Source: CAD feature listing. Evaluate the final solid. Frame: model axes, mm. A direction names the side the tool comes from. Give positions to 0.01 mm unless a question says otherwise; leave off trailing zeros. Order: outer loops, then holes, each group sorted by start corner. A loop starts at its lowest first (then second) coordinate and runs counter-clockwise, first axis right, second up. Notation, with made-up numbers: (62.5, 18) -> (81.5, 18) arc R25 cw to (81.5, 37) -> close; hole circle Ø4 at (-33, 62.5). An arc over 180 degrees is marked (long way). Answer in a Markdown table with one row per item.
Autodesk Inventor part; units mm, degrees
ref_plane "YZ Plane" through (0, 0, 0) normal (1, 0, 0) x (0, 1, 0)
ref_plane "XZ Plane" through (0, 0, 0) normal (0, 1, 0) x (-1, 0, 0)
ref_plane "XY Plane" through (0, 0, 0) normal (0, 0, 1) x (1, 0, 0)
sketch "Sketch1" plane through (0, 0, 0) normal (0, 0, 1) x (1, 0, 0)
  circle A0 centre (10.5, -1.5) radius 0.95
  circle A1 centre (-10.5, -1.5) radius 0.95
  line L0 (14, 9) -> (-14, 9)
  line L1 (-14, 9) -> (-14, -9)
  line L2 (-14, -9) -> (-7.5, -9)
  line L3 (-7.5, -9) -> (-7.5, -1.5)
  arc A2 (7.5, -1.5) -> (-7.5, -1.5) centre (0, -1.5) ccw
  line L4 (7.5, -1.5) -> (7.5, -9)
  line L5 (7.5, -9) -> (14, -9)
  line L6 (14, -9) -> (14, 9)
  line L7 (-7.5, -9) -> (7.5, -9)
  point P0 (0, 0)
extrude "Extrusion1" add sketch "Sketch1" along normal blind 3
sketch "Sketch2" plane through (0, 0, 3) normal (0, 0, 1) x (1, 0, 0)
  circle A0 centre (0, -1.5) radius 3
  circle A1 centre (0, -1.5) radius 2.95
  point P0 (0, 0)
  dimension "d4" = 5.9
extrude "Extrusion2" add sketch "Sketch2" along normal blind 5 contours A1
sketch "Sketch3" plane through (0, -1.5, 8) normal (0, 0, 1) x (1, 0, 0)
  circle A0 centre (0, 0) radius 2.95
  circle A1 centre (0, 0) radius 1.75
  point P0 (0, 1.5)
  dimension "d7" = 3.5
extrude "Extrusion3" cut sketch "Sketch3" against normal blind 8 contours A1
sketch "Sketch4" plane through (0, 0, 3) normal (0, 0, 1) x (1, 0, 0)
  circle A0 centre (0, -1.5) radius 2.95
  line L0 (14, -9) -> (14, 9)
  line L1 (14, 9) -> (-14, 9)
  line L2 (-14, 9) -> (-14, -9)
  line L3 (-14, -9) -> (14, -9)
  circle A1 centre (10.5, -1.5) radius 0.95
  circle A2 centre (-10.5, -1.5) radius 0.95
  line L4 (-5, -2) -> (-5, -1)
  line L5 (-5, -1) -> (5, -1)
  line L6 (5, -1) -> (5, -2)
  line L7 (5, -2) -> (-5, -2)
  line L8 (-5, -2) -> (5, -1) construction
  line L9 (-5, -1) -> (5, -2) construction
  point P0 (0, 0)
  dimension "d10" = 1
  dimension "d11" = 10
extrude "Extrusion4" cut sketch "Sketch4" along normal up to surface (5 mm away) contours A0 L7 L5 | A0 L5 L6 L7 | A0 L7 L4 L5
fillet "Fillet1" radius 0.5 4 edges at (2.2922, -2, 3) (-2.2922, -2, 3) (2.2922, -1, 3) (-2.2922, -1, 3)
sketch "Sketch5" plane through (0, 0, 3) normal (0, 0, 1) x (1, 0, 0)
  arc A0 (2.95, -1.5) -> (-2.95, -1.5) centre (0, -1.5) ccw
  arc A1 (-2.95, -1.5) -> (2.95, -1.5) centre (0, -1.5) ccw
  line L0 (14, -9) -> (14, 9)
  line L1 (14, 9) -> (-14, 9)
  line L2 (-14, 9) -> (-14, -9)
  line L3 (-14, -9) -> (14, -9)
  circle A2 centre (10.5, -1.5) radius 0.95
  circle A3 centre (-10.5, -1.5) radius 0.95
  line L4 (-17.5, -6.5) -> (-17.5, 3.5)
  line L5 (-17.5, 3.5) -> (17.5, 3.5)
  line L6 (17.5, 3.5) -> (17.5, -6.5)
  line L7 (17.5, -6.5) -> (-17.5, -6.5)
  line L8 (-17.5, -6.5) -> (17.5, 3.5) construction
  line L9 (-17.5, 3.5) -> (17.5, -6.5) construction
  point P0 (0, 0)
  point P1 (-14, 3.5)
  point P2 (14, 3.5)
  point P3 (14, -6.5)
  point P4 (-14, -6.5)
  dimension "d15" = 10
  dimension "d16" = 35
extrude "Extrusion5" cut sketch "Sketch5" against normal blind 8 contours L3 L2 L7 L0 | L5 L2 L1 L0
chamfer "Chamfer1" distance 2 angle 45 4 edges at (-14, 3.5, 1.5) (-14, -6.5, 1.5) (14, 3.5, 1.5) (14, -6.5, 1.5)
properties part number "pin_1"
(1) Ray query, probe 1 along Y at (x, z) = (10.5, 1.6); probe 2 along Y at (x, z) = (0, 1.75); probe 3 along X at (y, z) = (-2, 3.25). Return the intervals inside material, ascending.
A:
| item | result |
|---|---|
| probe 1 | y = -6.5 to -2.45, -0.55 to 3.5 |
| probe 2 | y = -6.5 to -3.25, 0.25 to 3.5 |
| probe 3 | x = -2.91 to -1.68, 1.68 to 2.91 |
(2) Access query for faces 1 (the flat face through (0, 1, 8)), 2 (the flat face through (-2, -2, 6)), 3 (the cylindrical face through (0.06, -4.45, 5.46)), 4 (the cylindrical face through (-0.06, 1.45, 5.46)). Directions: +Z, -Z, +X, -X, +Y, -Y. A direction counts if a zero-diameter tool reaches every point of the face in a straight line with its end or side. Return the directions, or none.
A:
| item | result |
|---|---|
| face 1 | +Z, +X, -X, +Y, -Y |
| face 2 | +Z, +X, -X |
| face 3 | +Z, -Y |
| face 4 | +Z, +Y |
(3) Pull-direction query (Y, two-part tool) for faces 5 (the flat face through (-2, -1, 6)), 6 (the flat face through (0, -3.5, 8)), 7 (the flat face through (-13, -5.5, 1.5)), 8 (the flat face through (2, -1, 6)); classes: +Y half, -Y half, draft (parallel to the pull), parting line (faces both ways), or undercut.
A:
| item | result |
|---|---|
| face 5 | undercut |
| face 6 | draft |
| face 7 | -Y half |
| face 8 | undercut |
(4) Section query C-C (z = 6). Return the cut outline in (x, y), plus the area to 3 significant figures.
A:
| item | result |
|---|---|
| outline | (-2.91, -2) arc R2.95 ccw to (2.91, -2) -> (1.68, -2) arc R1.75 cw to (-1.68, -2) -> close; (-2.91, -1) -> (-1.68, -1) arc R1.75 cw to (1.68, -1) -> (2.91, -1) arc R2.95 ccw to start |
| area | 15.3 mm^2 |
(5) Section query B-B (z = 2.5). Return the cut outline in (x, y), plus the area to 3 significant figures.
A:
| item | result |
|---|---|
| outline | (-14, -4.5) -> (-12, -6.5) -> (12, -6.5) -> (14, -4.5) -> (14, 1.5) -> (12, 3.5) -> (-12, 3.5) -> (-14, 1.5) -> close; hole circle Ø1.9 at (-10.5, -1.5); hole circle Ø3.5 at (0, -1.5); hole circle Ø1.9 at (10.5, -1.5) |
| area | 257 mm^2 |
(6) Section query A-A (x = 10.5). Return the cut outline in (y, z), plus the area to 3 significant figures.
A:
| item | result |
|---|---|
| outline | (-6.5, 0) -> (-2.45, 0) -> (-2.45, 3) -> (-6.5, 3) -> close; (-0.55, 0) -> (3.5, 0) -> (3.5, 3) -> (-0.55, 3) -> close |
| area | 24.3 mm^2 |
(7) Section query D-D (y = -2.75). Return the cut outline in (x, z).
A:
| item | result |
|---|---|
| outline | (-14, 0) -> (-1.22, 0) -> (-1.22, 8) -> (-2.67, 8) -> (-2.67, 3) -> (-14, 3) -> close; (1.22, 0) -> (14, 0) -> (14, 3) -> (2.67, 3) -> (2.67, 8) -> (1.22, 8) -> close |
(8) First-contact query: pin 1 Ø5.5 at (x, y) = (0, -1.5) entering from +Z; pin 2 Ø1.5 at (x, y) = (-10.5, -1.5) entering from +Z; pin 3 Ø1.4 at (x, z) = (-2.5, 6) entering from +Y; pin 4 Ø1 at (x, z) = (2.5, 5) entering from -Y. Flat tips, straight axial feed; report the tip coordinate or a pass-through.
A:
| item | result |
|---|---|
| pin 1 | stops at z = 8 |
| pin 2 | passes through |
| pin 3 | stops at y = 0.84 |
| pin 4 | stops at y = -3.67 |
